Work out the finished part from the listing and answer in its coordinate system (mm). A direction names the side the tool comes from. Give positions to 0.01 mm unless a question says otherwise; leave off trailing zeros. Loops run counter-clockwise (first coordinate to the right, second up) from the corner with the lowest first, then second, coordinate; pieces in that order, holes last. Notation, with made-up numbers: (-14.5, 36) - (6.5, 36) arc R11 ccw to (6.5, 50) - close; hole circle Ø3 at (74, 20). An arc over 180 degrees is marked (long way). One line per item, written item: value.
from build123d import *

# Parameters (mm, degrees)
F0_R     = 10.16
F1_DEPTH = 15.7734
F3_DEPTH = 24.4602
F4_SIZE  = 3.302


with BuildPart() as f1:
    # F0 (on Top) → F1 (new body)
    with BuildSketch(Plane.XY):
        with BuildLine():
            ThreePointArc((5.0426470588, -28.1265414802), (21.9160245563, -18.3362616868), (28.575, 0))
            ThreePointArc((28.575, 0), (21.9160245563, 18.3362616868), (5.0426470588, 28.1265414802))
            ThreePointArc((5.0426470588, 28.1265414802), (-28.575, 0), (5.0426470588, -28.1265414802))
        make_face()
        with BuildLine():
            ThreePointArc((-13.4477648793, 4.826), (0, 14.2875), (13.4477648793, 4.826))
            Line((13.4477648793, 4.826), (16.4084, 4.826))
            Line((16.4084, 4.826), (16.4084, -4.826))
            Line((16.4084, -4.826), (13.4477648793, -4.826))
            ThreePointArc((13.4477648793, -4.826), (0, -14.2875), (-13.4477648793, -4.826))
            Line((-13.4477648793, -4.826), (-16.4084, -4.826))
            Line((-16.4084, -4.826), (-16.4084, 4.826))
            Line((-16.4084, 4.826), (-13.4477648793, 4.826))
        make_face(mode=Mode.SUBTRACT)
        with BuildLine():
            ThreePointArc((5.0426470588, 28.1265414802), (21.9160245563, 18.3362616868), (28.575, 0))
            ThreePointArc((28.575, 0), (21.9160245563, -18.3362616868), (5.0426470588, -28.1265414802))
            Line((5.0426470588, -28.1265414802), (57.3367647059, -18.7510276535))
            ThreePointArc((57.3367647059, -18.7510276535), (34.925, 0), (57.3367647059, 18.7510276535))
            Line((57.3367647059, 18.7510276535), (5.0426470588, 28.1265414802))
        make_face()
        with BuildLine():
            ThreePointArc((73.025, 0), (68.5856830375, 12.2241744579), (57.3367647059, 18.7510276535))
            ThreePointArc((57.3367647059, 18.7510276535), (34.925, 0), (57.3367647059, -18.7510276535))
            ThreePointArc((57.3367647059, -18.7510276535), (68.5856830375, -12.2241744579), (73.025, 0))
        make_face()
        with Locations((53.975, 0)):
            Circle(F0_R, mode=Mode.SUBTRACT)
        with BuildLine():
            ThreePointArc((-13.4477648793, -4.826), (-14.2875, 0), (-13.4477648793, 4.826))
            Line((-13.4477648793, 4.826), (-16.4084, 4.826))
            Line((-16.4084, 4.826), (-16.4084, -4.826))
            Line((-16.4084, -4.826), (-13.4477648793, -4.826))
        make_face()
    extrude(amount=F1_DEPTH)

    # F2 (on face) → F3 (join)
    with BuildSketch(Plane.XY.offset(15.7734)):
        with BuildLine():
            ThreePointArc((5.0426470588, -28.1265414802), (21.9160245563, -18.3362616868), (28.575, 0))
            ThreePointArc((28.575, 0), (21.9160245563, 18.3362616868), (5.0426470588, 28.1265414802))
            ThreePointArc((5.0426470588, 28.1265414802), (-28.575, 0), (5.0426470588, -28.1265414802))
        make_face()
        with BuildLine():
            ThreePointArc((13.4477648793, -4.826), (-14.2875, 0), (13.4477648793, 4.826))
            Line((13.4477648793, 4.826), (16.4084, 4.826))
            Line((16.4084, 4.826), (16.4084, -4.826))
            Line((16.4084, -4.826), (13.4477648793, -4.826))
        make_face(mode=Mode.SUBTRACT)
    extrude(amount=F3_DEPTH)

    # F4
    f4_edges = [f1.edges().sort_by_distance(p)[0] for p in [
        (-5.042647, 28.126541, 40.2336),
    ]]
    chamfer(f4_edges, length=F4_SIZE)


solid = f1.part
1. Flat-ended cylindrical pins translate along their axes: pin 1 Ø5 at (x, y) = (34.5, -12.5) entering from -Z; pin 2 Ø1.5 at (x, z) = (-10, 31.5) entering from -Y; pin 3 Ø5 at (x, z) = (40, 10) entering from +Y; pin 4 Ø1.5 at (x, z) = (48, 18) entering from +Y. Find the tip coordinate at first contact, or state that the pin passes through.
Output:
pin 1: stops at z = 0
pin 2: stops at y = -27.04
pin 3: stops at y = 22.31
pin 4: passes through
2. Find the intervals of material crossed by line 1 along X through (y, z) = (0, 31.25) (1 decimal); line 2 along X through (y, z) = (-7, 12); line 3 along Z through (x, y) = (36, -1.5), in increasing order.
Output:
line 1: x = -28.6 to -14.3, 16.4 to 28.6
line 2: x = -27.7 to -12.46, 12.46 to 46.61, 61.34 to 71.69
line 3: z = 0 to 15.77
3. Section A-A (x = 0) is taken. Write down the section's boundary in (y, z) (1 decimal), and give its area (3 significant figures).
Output:
outline: (-28.6, 0) - (-14.3, 0) - (-14.3, 40.2) - (-25.3, 40.2) - (-28.6, 36.9) - close; (14.3, 0) - (28.6, 0) - (28.6, 36.9) - (25.3, 40.2) - (14.3, 40.2) - close
area: 1,140 mm²
4. Section C-C (x = 60.5) is taken. Write down the section's boundary in (y, z).
Output:
outline: (-17.9, 0) - (-7.79, 0) - (-7.79, 15.77) - (-17.9, 15.77) - close; (7.79, 0) - (17.9, 0) - (17.9, 15.77) - (7.79, 15.77) - close
5. Section D-D (y = 2.5) is taken. Count the separate pieces of the cut face and the enclosed holes in it, and give its area (3 significant figures).
Output:
separate pieces: 3
enclosed holes: 0
area: 1,440 mm²
6. The mould has two halves that part along Y. Classify faces 1 (the flat face through (22, 0, 0)), 2 (the flat face through (16.408, 0, 20)), 3 (the flat face through (31.556, 23.373, 7.776)): released by +Y, released by -Y, zero draft, split by the parting line, or undercut.
Output:
face 1: zero draft
face 2: undercut
face 3: released by +Y
7. For faces 4 (the flat face through (15, 4.826, 20)), 5 (the flat face through (11, -11, 40.234)), determine the directions among +Z, -Z, +X, -X, +Y, -Y from which every point of the face is accessible in a straight line to the end or side of a thin tool.
Output:
face 4: +Z, -Z
face 5: +Z, +X, -X, +Y, -Y
